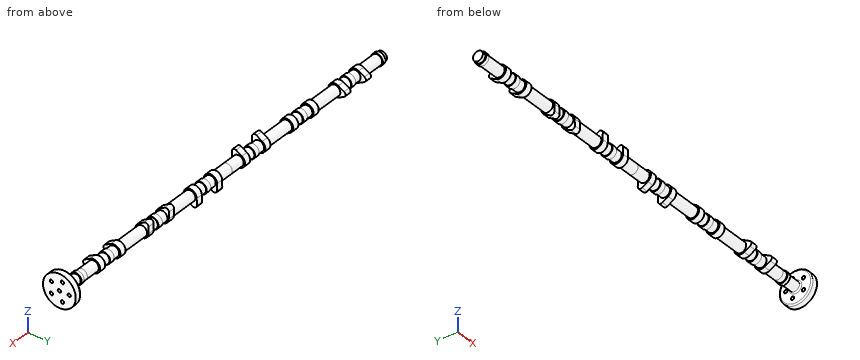
```python
from build123d import *
from build123d.topology import SkipClean

# Parameters (mm, degrees)
SKETCH1_R             = 8
BOSS_EXTRUDE1_DEPTH   = 47.5
BOSS_EXTRUDE2_START   = 15
BOSS_EXTRUDE2_DEPTH   = 10
SKETCH3_R             = 9
BOSS_EXTRUDE3_DEPTH   = 4
LPATTERN1_COUNT       = 6
LPATTERN1_PITCH       = 95
BODY_MOVE_COPY1_ANGLE = 60
BODY_MOVE_COPY2_ANGLE = 120
BODY_MOVE_COPY3_ANGLE = 60
BODY_MOVE_COPY4_ANGLE = 120
BODY_MOVE_COPY5_ANGLE = 180
SKETCH4_R             = 8
BOSS_EXTRUDE4_DEPTH   = 10
SKETCH5_R             = 9
BOSS_EXTRUDE5_DEPTH   = 5
SKETCH6_R             = 7.5
BOSS_EXTRUDE6_DEPTH   = 5
SKETCH7_R             = 8
BOSS_EXTRUDE7_DEPTH   = 7.5
SKETCH8_R             = 9
BOSS_EXTRUDE8_DEPTH   = 5
SKETCH9_R             = 7.5
BOSS_EXTRUDE9_DEPTH   = 22.3
SKETCH10_R            = 25
SKETCH10_R_2          = 2.5
BOSS_EXTRUDE10_DEPTH  = 10
SKETCH11_R            = 2.5
CUT_EXTRUDE1_DEPTH    = 15
FILLET1_R             = 2


with BuildPart() as part:
    # Sketch1 → Boss-Extrude1 (new, symmetric)
    with BuildSketch(Plane(origin=(0, 0, 0), x_dir=(0, 0, -1), z_dir=(1, 0, 0))):
        Circle(SKETCH1_R)
    extrude(amount=BOSS_EXTRUDE1_DEPTH, both=True)

    # Sketch2 → Boss-Extrude2 (add)
    with BuildSketch(Plane(origin=(0, 0, 0), x_dir=(0, 0, -1), z_dir=(1, 0, 0)).offset(BOSS_EXTRUDE2_START)):
        with BuildLine():
            Line((-8.746197071, -4.848096202), (-3.807936598, -13.756953924))
            ThreePointArc((-3.807936598, -13.756953924), (0, -16), (3.807936598, -13.756953924))
            Line((3.807936598, -13.756953924), (8.746197071, -4.848096202))
            ThreePointArc((8.746197071, -4.848096202), (0, 10), (-8.746197071, -4.848096202))
        make_face()
    boss_extrude2 = extrude(amount=BOSS_EXTRUDE2_DEPTH)

    # Mirror1: Boss-Extrude2 across plane
    add(boss_extrude2.mirror(Plane(origin=(0, 0, 0), x_dir=(0, 0, 1), z_dir=(1, 0, 0))))

    # Sketch3 → Boss-Extrude3 (add, symmetric)
    with BuildSketch(Plane(origin=(0, 0, 0), x_dir=(0, 0, -1), z_dir=(1, 0, 0))):
        Circle(SKETCH3_R)
    extrude(amount=BOSS_EXTRUDE3_DEPTH, both=True)


with BuildPart() as lpattern1_1:
    # LPattern1: pattern copy
    add(part.part.moved(Location(Vector(-1, 0, 0) * (1 * LPATTERN1_PITCH))))


with BuildPart() as lpattern1_2:
    # LPattern1: pattern copy
    add(part.part.moved(Location(Vector(-1, 0, 0) * (2 * LPATTERN1_PITCH))))


with BuildPart() as lpattern1_3:
    # LPattern1: pattern copy
    add(part.part.moved(Location(Vector(-1, 0, 0) * (3 * LPATTERN1_PITCH))))


with BuildPart() as lpattern1_4:
    # LPattern1: pattern copy
    add(part.part.moved(Location(Vector(-1, 0, 0) * (4 * LPATTERN1_PITCH))))


with BuildPart() as lpattern1_5:
    # LPattern1: pattern copy
    add(part.part.moved(Location(Vector(-1, 0, 0) * (5 * LPATTERN1_PITCH))))


with BuildPart() as lpattern1_3_1:
    # Body-Move_Copy1: moved
    add(lpattern1_3.part.rotate(Axis((0, 0, 0), (-1, 0, 0)), BODY_MOVE_COPY1_ANGLE))


with BuildPart() as lpattern1_1_1:
    # Body-Move_Copy2: moved
    add(lpattern1_1.part.rotate(Axis((0, 0, 0), (-1, 0, 0)), BODY_MOVE_COPY2_ANGLE))


with BuildPart() as lpattern1_4_1:
    # Body-Move_Copy3: moved
    add(lpattern1_4.part.rotate(Axis((0, 0, 0), (1, 0, 0)), BODY_MOVE_COPY3_ANGLE))


with BuildPart() as lpattern1_2_1:
    # Body-Move_Copy4: moved
    add(lpattern1_2.part.rotate(Axis((0, 0, 0), (1, 0, 0)), BODY_MOVE_COPY4_ANGLE))


with BuildPart() as lpattern1_5_1:
    # Body-Move_Copy5: moved
    add(lpattern1_5.part.rotate(Axis((0, 0, 0), (1, 0, 0)), BODY_MOVE_COPY5_ANGLE))

    # Sketch4 → Boss-Extrude4 (add)
    with BuildSketch(Plane.ZY.offset(522.5)):
        Circle(SKETCH4_R)
    extrude(amount=BOSS_EXTRUDE4_DEPTH)

    # Sketch5 → Boss-Extrude5 (add)
    with BuildSketch(Plane.ZY.offset(532.5)):
        Circle(SKETCH5_R)
    extrude(amount=BOSS_EXTRUDE5_DEPTH)


with BuildPart() as lpattern1_4_2:
    add(lpattern1_4_1.part)

    # Combine1: union LPattern1_1, LPattern1_3, LPattern1_2, part, LPattern1_5
    add(lpattern1_1_1.part)
    add(lpattern1_3_1.part)
    add(lpattern1_2_1.part)
    add(part.part)
    add(lpattern1_5_1.part)

    # Sketch6 → Boss-Extrude6 (add)
    with BuildSketch(Plane.ZY.offset(537.5)):
        Circle(SKETCH6_R)
    extrude(amount=BOSS_EXTRUDE6_DEPTH)

    # Sketch7 → Boss-Extrude7 (add)
    with SkipClean():  # the faces are left unmerged after this step: merging them gives an invalid solid
        with BuildSketch(Plane(origin=(47.5, 0, 0), x_dir=(0, 0, -1), z_dir=(1, 0, 0))):
            with Locations(Location((0, 0, 0), (0, 0, 60))):
                Circle(SKETCH7_R)
        extrude(amount=BOSS_EXTRUDE7_DEPTH)
    add(lpattern1_4_2.part.scale(1), mode=Mode.REPLACE)  # the faces are merged on a copy

    # Sketch8 → Boss-Extrude8 (add)
    with SkipClean():  # the faces are left unmerged after this step: merging them gives an invalid solid
        with BuildSketch(Plane(origin=(55, 0, 0), x_dir=(0, 0, -1), z_dir=(1, 0, 0))):
            with Locations(Location((0, 0, 0), (0, 0, 60))):
                Circle(SKETCH8_R)
        extrude(amount=BOSS_EXTRUDE8_DEPTH)

    # Sketch9 → Boss-Extrude9 (add)
    with SkipClean():  # the faces are left unmerged after this step: merging them gives an invalid solid
        with BuildSketch(Plane(origin=(60, 0, 0), x_dir=(0, 0, -1), z_dir=(1, 0, 0))):
            with Locations(Location((0, 0, 0), (0, 0, 180))):
                Circle(SKETCH9_R)
        extrude(amount=BOSS_EXTRUDE9_DEPTH)

    # Sketch10 → Boss-Extrude10 (add)
    with SkipClean():  # the faces are left unmerged after this step: merging them gives an invalid solid
        with BuildSketch(Plane(origin=(82.3, 0, 0), x_dir=(0, 0, -1), z_dir=(1, 0, 0))):
            Circle(SKETCH10_R)
            Circle(SKETCH10_R_2, mode=Mode.SUBTRACT)
        extrude(amount=BOSS_EXTRUDE10_DEPTH)

    # Sketch11 → Cut-Extrude1 (cut)
    with SkipClean():  # the faces are left unmerged after this step: merging them gives an invalid solid
        with BuildSketch(Plane(origin=(92.3, 0, 0), x_dir=(0, 0, -1), z_dir=(1, 0, 0))):
            with Locations((0, 15)):
                Circle(SKETCH11_R)
            Circle(SKETCH11_R)
            with Locations((14.265847744, 4.635254916)):
                Circle(SKETCH11_R)
            with Locations((8.816778784, -12.135254916)):
                Circle(SKETCH11_R)
            with Locations((-8.816778784, -12.135254916)):
                Circle(SKETCH11_R)
            with Locations((-14.265847744, 4.635254916)):
                Circle(SKETCH11_R)
        extrude(amount=-CUT_EXTRUDE1_DEPTH, mode=Mode.SUBTRACT)

    # Fillet1
    fillet1_edges = [lpattern1_4_2.edges().sort_by_distance(p)[0] for p in [
        (82.3, 0, -7.5),
        (82.3, 0, 25),
    ]]
    fillet(fillet1_edges, radius=FILLET1_R)


solid = lpattern1_4_2.part
```
Design review of the part built by this model. Coordinates are the model's own, in mm. Coordinates: 2 decimals unless noted, no trailing zeros. Order: outer loops, then holes, each group sorted by start corner. A loop starts at its lowest first (then second) coordinate and runs counter-clockwise, first axis right, second up.
1) Wall thickness on line 1 along Y through (x, z) = (85.75, 0); line 2 along Y through (x, z) = (-182, 0.5); line 3 along X through (y, z) = (13, 16.5): over which ranges is each line inside the solid? List them lowest first.
2) Clearance check with flat-ended pins moving along their axes: pin 1 (6.5 mm diameter, centred on y = 0, z = 0, fed in from +X); pin 2 (3 mm diameter, centred on y = 4.64, z = -14.27, fed in from +X); pin 3 (12 mm diameter, centred on x = -327.5, y = -1, fed in from +Z); pin 4 (1.5 mm diameter, centred on x = -345, z = -9, fed in from -Y). State where each tip first meets the part, or that it passes through.
3) Take a section at A-A, the plane x = 37. Give the boundary of the cut face in (y, z), and give its area (3 significant figures).
Returned:
1. line 1: y = -25 to -2.5, 2.5 to 12.5, 17.5 to 25
1. line 2: y = -7.98 to 7.98
1. line 3: x = 82.3 to 92.3
2. pin 1: stops at x = 92.3
2. pin 2: stops at x = -165
2. pin 3: stops at z = 8
2. pin 4: passes through
3. outline: circle Ø16 at (0, 0)
3. area: 201 mm2
